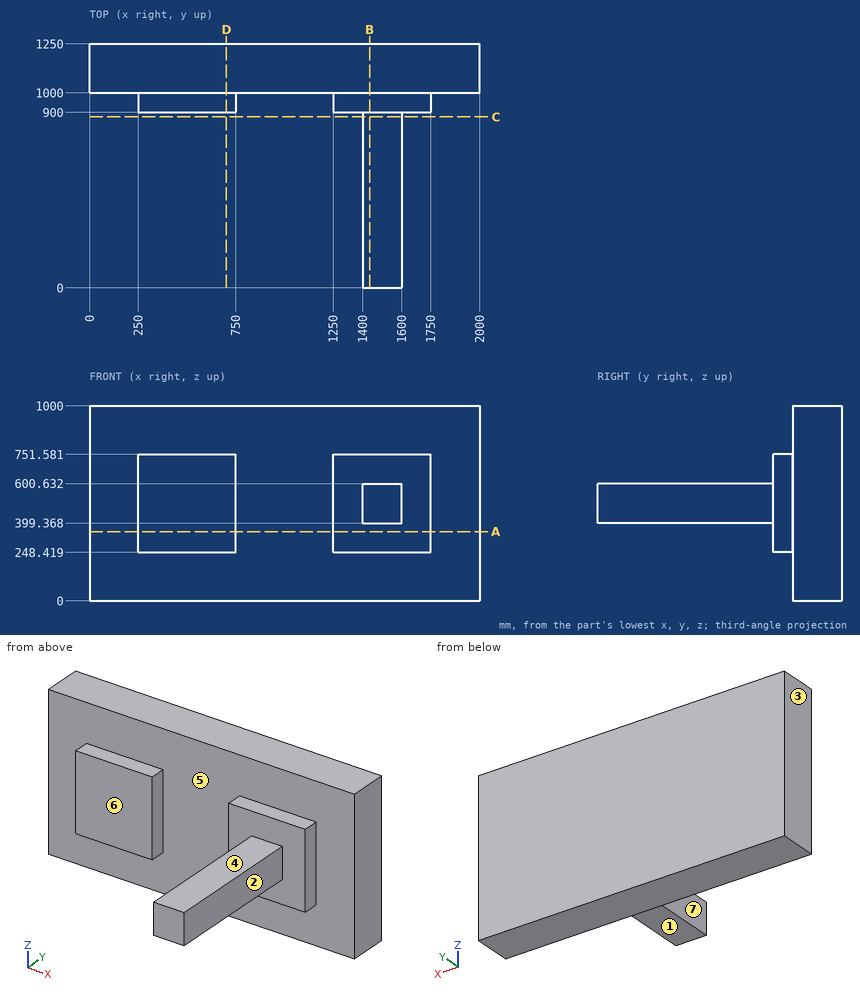
Geometry check sheet. Reference: drawing and pictorial views, mm from the part's lowest x, y, z. A direction names the side the tool comes from. Round coordinates to 2 decimals unless told otherwise and drop trailing zeros. Loops run counter-clockwise (first coordinate to the right, second up) from the corner with the lowest first, then second, coordinate; pieces in that order, holes last.
1. Sectioned sample at A-A on z = 355. Record the boundary of the cut face in (x, y), and give its area (3 significant figures).
2. Mould release check, pull along X, two halves, no side actions. Record for the marked faces 5, 6 and 7: released by +X, released by -X, zero draft, split by the parting line, or undercut.
3. Scan lines: probe 1 along Y at (x, z) = (1192, 523); probe 2 along X at (y, z) = (659.5, 478); probe 3 along Y at (x, z) = (646, 260). Record each from-to range of solid material in increasing order.
4. Gauge pin test, flat ends, axial feed: pin 1 Ø5 at (x, y) = (325, 978.5) entering from +Z; pin 2 Ø4 at (x, z) = (1277, 165.5) entering from -Y. Record the tip position at first contact, or that the pin passes through.
5. Sectioned sample at D-D on x = 702. Record the boundary of the cut face in (y, z), and give its area (3 significant figures).
6. Sectioned sample at B-B on x = 1436. Record the boundary of the cut face in (y, z).
7. Set-up check for the marked faces 1, 2, 3 and 4: record each of +Z, -Z, +X, -X, +Y, -Y from which the full face is reachable in a straight line by a thin tool's end or side.
8. Sectioned sample at C-C on y = 877. Record the boundary of the cut face in (x, z), and give its area (3 significant figures).
Recorded:
1. outline: (0, 1000) - (250, 1000) - (250, 900) - (750, 900) - (750, 1000) - (1250, 1000) - (1250, 900) - (1750, 900) - (1750, 1000) - (2000, 1000) - (2000, 1250) - (0, 1250) - close
1. area: 600,000 mm2
2. face 5: undercut
2. face 6: zero draft
2. face 7: released by -X
3. probe 1: y = 1000 to 1250
3. probe 2: x = 1400 to 1600
3. probe 3: y = 900 to 1250
4. pin 1: stops at z = 751.58
4. pin 2: stops at y = 1000
5. outline: (900, 248.42) - (1000, 248.42) - (1000, 0) - (1250, 0) - (1250, 1000) - (1000, 1000) - (1000, 751.58) - (900, 751.58) - close
5. area: 300,000 mm2
6. outline: (0, 399.37) - (900, 399.37) - (900, 248.42) - (1000, 248.42) - (1000, 0) - (1250, 0) - (1250, 1000) - (1000, 1000) - (1000, 751.58) - (900, 751.58) - (900, 600.63) - (0, 600.63) - close
7. face 1: -Z, +X, -X, -Y
7. face 2: +Z, -Z, +X, -Y
7. face 3: +Z, -Z, -X, +Y, -Y
7. face 4: +Z, +X, -X, -Y
8. outline: (1400, 399.37) - (1600, 399.37) - (1600, 600.63) - (1400, 600.63) - close
8. area: 40,300 mm2
